Here's the drawing with two shaded views (mm, measured from the low corner). I have some questions. Coordinates: 2 decimals unless noted, no trailing zeros. Write each loop counter-clockwise with the first axis right and the second up, starting at its lowest first coordinate (ties: lowest second). Pieces come first, ordered by that corner, then holes.
Item 1: I want a section at B-B on y = 17.5. Please give me the cut outline in (x, z), then the cut area to 3 significant figures.
Item 2: Thinking about a two-plate mould opening in Z: for the marked faces 1, 2 and 3, which applies, +Z half, -Z half, draft (parallel to the pull), parting line (faces both ways), or undercut?
Item 3: I want a section at A-A on z = 57.15. Please give me the cut outline in (x, y) (3 decimals), then the cut area to 3 significant figures.
Item 4: For P1, Ø1.9, axis at x = 7.5, y = 24, coming from the -Z side, with a flat end and sliding along its axis, tell me the tip position at first contact or that it passes through.
Item 5: If I drill on probe 1 along Y at (x, z) = (6.35, 14.5) (3 decimals); probe 2 along Y at (x, z) = (1, 57.5); probe 3 along Y at (x, z) = (9.25, 13.5), over which ranges is the centre line in solid material (lowest first)?
Item 6: I want a section at D-D on x = 10.75. Please give me the cut outline in (y, z) (3 decimals), then the cut area to 3 significant figures.
Item 7: I want a section at C-C on y = 6.35. Please give me the cut outline in (x, z) (3 decimals).
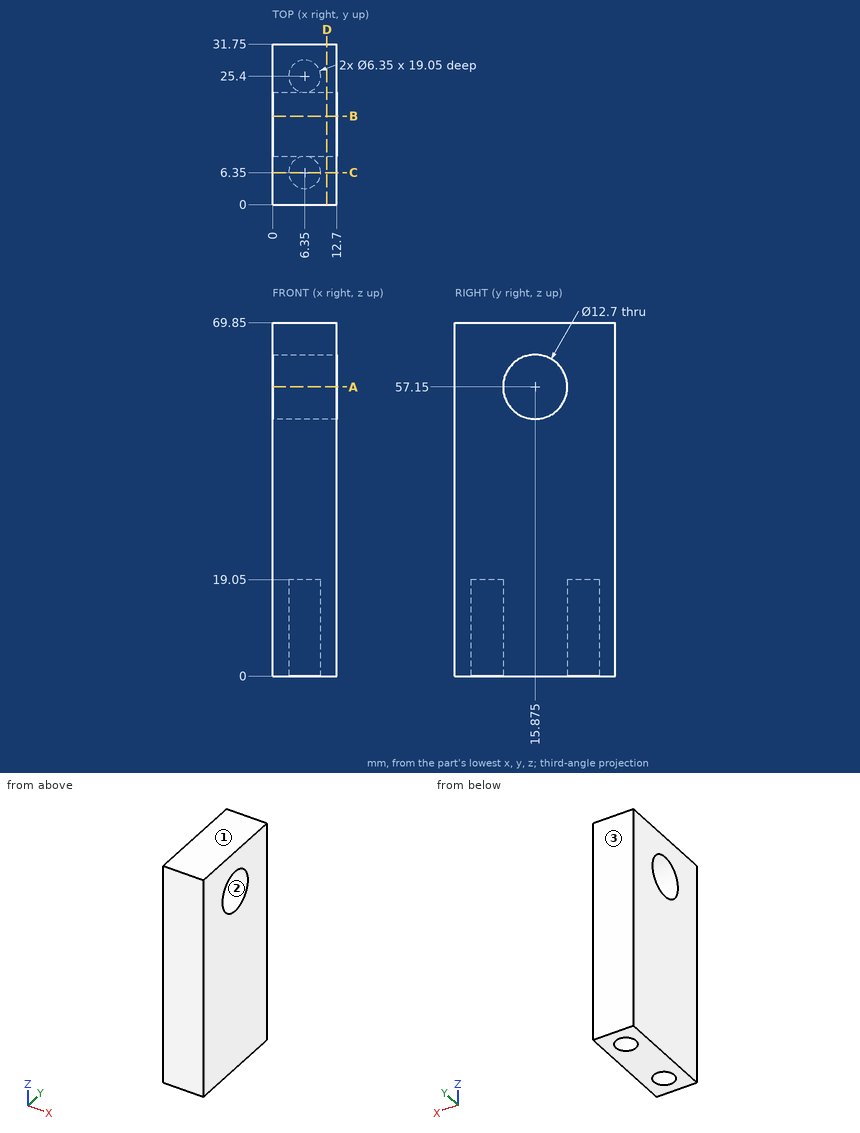
Response values:
1. outline: (0, 0) - (12.7, 0) - (12.7, 51.01) - (0, 51.01) - close; (0, 63.29) - (12.7, 63.29) - (12.7, 69.85) - (0, 69.85) - close
1. area: 731 mm2
2. face 1: +Z half
2. face 2: undercut
2. face 3: draft
3. outline: (0, 0) - (12.7, 0) - (12.7, 9.525) - (0, 9.525) - close; (0, 22.225) - (12.7, 22.225) - (12.7, 31.75) - (0, 31.75) - close
3. area: 242 mm2
4. P1: stops at z = 19.05
5. probe 1: y = 0 to 3.175, 9.525 to 22.225, 28.575 to 31.75
5. probe 2: y = 0 to 9.53, 22.22 to 31.75
5. probe 3: y = 0 to 5.06, 7.64 to 24.11, 26.69 to 31.75
6. outline: (0, 0) - (31.75, 0) - (31.75, 69.85) - (0, 69.85) - close; hole circle Ø12.7 at (15.875, 57.15)
6. area: 2,090 mm2
7. outline: (0, 0) - (3.175, 0) - (3.175, 19.05) - (9.525, 19.05) - (9.525, 0) - (12.7, 0) - (12.7, 69.85) - (0, 69.85) - close
